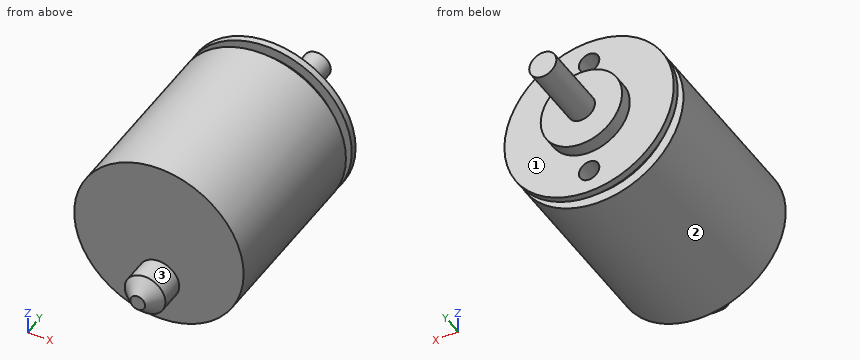
```python
from build123d import *

# Parameters (mm, degrees)
F0_W     = 2
F0_H     = 10
F3_D     = 3
F3_DEPTH = 4
F3_TIP   = 0.9012909285
F4_R     = 3
F5_DEPTH = 5.5
F6_SIZE  = 1.905


with BuildPart() as f1:
    # F0 (on Top) → F1 (revolve)
    with BuildSketch(Plane.XY):
        Polygon((6, 29), (0, 29), (0, 0), (12.5, 0), (12.5, 26.5), (11, 26.5), (11, 28), (12.5, 28), (12.5, 29), align=None)
        Polygon((0, 31), (0, 29), (6, 29), (6, 31), (2, 31), align=None)
        with Locations((1, 36)):
            Rectangle(F0_W, F0_H)
    revolve(axis=Axis((0, 14.5, 0), (0, -1, 0)))

    # F3
    with Locations(Plane(origin=(0, 29, 0), x_dir=(-1, 0, 0), z_dir=(0, 1, 0))):
        with Locations((0, 9), (0, -9)):
            Hole(F3_D / 2, depth=F3_DEPTH)
            with Locations((0, 0, -(F3_DEPTH + F3_TIP / 2))):  # 118° drill point
                Cone(0, F3_D / 2, F3_TIP, mode=Mode.SUBTRACT)

    # F4 (on face) → F5 (join)
    with BuildSketch(Plane.XZ):
        with Locations((0, -6)):
            Circle(F4_R)
    extrude(amount=F5_DEPTH)

    # F6
    f6_edges = [f1.edges().sort_by_distance(p)[0] for p in [
        (-3, -5.5, -6),
    ]]
    chamfer(f6_edges, length=F6_SIZE)


solid = f1.part
```
Work out the finished part from the listing and answer in its coordinate system (mm). Face numbers are marked on the shaded views. A direction names the side the tool comes from. Give positions to 0.01 mm unless a question says otherwise; leave off trailing zeros. Loops run counter-clockwise (first coordinate to the right, second up) from the corner with the lowest first, then second, coordinate; pieces in that order, holes last. Notation, with made-up numbers: (-14, 71.5) -> (13, 71.5) arc R10 cw to (13, 83.5) -> close; hole circle Ø2 at (-39.5, 34.5). An arc over 180 degrees is marked (long way). Use CSV: the item, a comma, the result in double quotes.
1. Flat-ended cylindrical pins translate along their axes: pin 1 Ø4 at (x, z) = (8.5, 0) entering from +Y; pin 2 Ø1 at (x, z) = (4, 2.5) entering from +Y; pin 3 Ø2 at (x, y) = (7, 29.5) entering from +Z; pin 4 Ø12 at (x, z) = (-5, -5) entering from -Y. Find the tip coordinate at first contact, or state that the pin passes through.
Found:
pin 1,"y = 29"
pin 2,"y = 31"
pin 3,"z = 10.89"
pin 4,"y = -5.5"
2. Straight lines are drawn through the part: line 1 (Z direction, x = 0, y = 27.35); line 2 (Z direction, x = 0, y = 26.2); line 3 (Y direction, x = 7.75, z = -8.25). For each, find the intervals that lie inside material, in ascending order.
Found:
line 1,"-11 to -10.5, -7.5 to 7.5, 10.5 to 11"
line 2,"-12.5 to -10.5, -7.5 to 7.5, 10.5 to 12.5"
line 3,"0 to 26.5, 28 to 29"
3. The part is cut by section B-B (y = 26). Write down the section's boundary in (x, z).
Found:
outline,"circle Ø25 at (0, 0); hole circle Ø3 at (0, -9); hole circle Ø3 at (0, 9)"
4. The part is cut by section D-D (y = 38). Write down the section's boundary in (x, z), then the cut area to 3 significant figures.
Found:
outline,"circle Ø4 at (0, 0)"
area,"12.6 mm^2"
5. The part is cut by section C-C (x = 5.5). Write down the section's boundary in (y, z), then the cut area to 3 significant figures.
Found:
outline,"(0, -11.22) -> (26.5, -11.22) -> (26.5, -9.53) -> (28, -9.53) -> (28, -11.22) -> (29, -11.22) -> (29, -2.4) -> (31, -2.4) -> (31, 2.4) -> (29, 2.4) -> (29, 11.22) -> (28, 11.22) -> (28, 9.53) -> (26.5, 9.53) -> (26.5, 11.22) -> (0, 11.22) -> close"
area,"656 mm^2"
6. The part is cut by section A-A (z = 0). Write down the section's boundary in (x, y), then the cut area to 4 significant figures.
Found:
outline,"(-12.5, 0) -> (12.5, 0) -> (12.5, 26.5) -> (11, 26.5) -> (11, 28) -> (12.5, 28) -> (12.5, 29) -> (6, 29) -> (6, 31) -> (2, 31) -> (2, 41) -> (-2, 41) -> (-2, 31) -> (-6, 31) -> (-6, 29) -> (-12.5, 29) -> (-12.5, 28) -> (-11, 28) -> (-11, 26.5) -> (-12.5, 26.5) -> close"
area,"784.5 mm^2"
7. A tool of negligible diameter and unlimited length cuts with its end or side. For the marked faces 1, 2 and 3, from which of +Z, -Z, +X, -X, +Y, -Y can it reach the whole face along a straight path? Write none if from no direction.
Found:
face 1,"+Y"
face 2,"+Y, -Y"
face 3,"-Y"
